from build123d import *

# Parameters (mm, degrees)
CROQUIS1_W              = 60
CROQUIS1_H              = 120
SALIENTE_EXTRUIR1_DEPTH = 50
CROQUIS2_R              = 11
SALIENTE_EXTRUIR2_DEPTH = 8
CROQUIS3_R              = 10
CORTAR_EXTRUIR1_DEPTH   = 0.1
SALIENTE_EXTRUIR3_DEPTH = 0.1
CROQUIS5_R              = 5.530403268
CROQUIS5_R_2            = 4.15467208
SALIENTE_EXTRUIR4_DEPTH = 0.1
REDONDEO1_R             = 2
CROQUIS6_R              = 9
SALIENTE_EXTRUIR5_DEPTH = 10
CHAFL_N1_SIZE           = 3
CHAFL_N1_SIZE2          = 2.100622615
CROQUIS8_R              = 6.899377385


with BuildPart() as part:
    # Croquis1 → Saliente-Extruir1 (new body)
    with BuildSketch(Plane.XY):
        with Locations((30, 60)):
            Rectangle(CROQUIS1_W, CROQUIS1_H)
    extrude(amount=SALIENTE_EXTRUIR1_DEPTH)

    # Croquis2 → Saliente-Extruir2 (add)
    with BuildSketch(Plane.XY.offset(50)):
        with Locations(Location((30, 60, 0), (0, 0, 180))):
            Circle(CROQUIS2_R)
        with Locations(Location((30, 90, 0), (0, 0, 180))):
            Circle(CROQUIS2_R)
        with Locations(Location((30, 30, 0), (0, 0, 180))):
            Circle(CROQUIS2_R)
    extrude(amount=SALIENTE_EXTRUIR2_DEPTH)

    # Croquis3 → Cortar-Extruir1 (cut)
    with BuildSketch(Plane.XY.offset(58)):
        with Locations((30, 90)):
            Circle(CROQUIS3_R)
        with Locations((30, 60)):
            Circle(CROQUIS3_R)
        with Locations((30, 30)):
            Circle(CROQUIS3_R)
    extrude(amount=-CORTAR_EXTRUIR1_DEPTH, mode=Mode.SUBTRACT)

    # Croquis4 → Saliente-Extruir3 (add)
    with BuildSketch(Plane.XY.offset(57.9)):
        Polygon((29.277033543, 82.393028635), (31.097592421, 82.393028635), (31.097592421, 93.369086775), (32.121534281, 93.369086775), (31.097592421, 94.393028635), (30.187312982, 95.303308074), (29.277033543, 94.393028635), (28.253091683, 93.369086775), (29.277033543, 93.369086775), align=None)
        Polygon((29.277033543, 26.630913225), (28.253091683, 26.630913225), (29.277033543, 25.606971365), (30.187312982, 24.696691926), (31.097592421, 25.606971365), (32.121534281, 26.630913225), (31.097592421, 26.630913225), (31.097592421, 37.606971365), (29.277033543, 37.606971365), align=None)
    extrude(amount=SALIENTE_EXTRUIR3_DEPTH)

    # Croquis5 → Saliente-Extruir4 (add)
    with BuildSketch(Plane.XY.offset(57.9)):
        with Locations((30, 60)):
            Circle(CROQUIS5_R)
        with Locations((30, 60)):
            Circle(CROQUIS5_R_2, mode=Mode.SUBTRACT)
    extrude(amount=SALIENTE_EXTRUIR4_DEPTH)

    # Redondeo1
    redondeo1_edges = [part.edges().sort_by_distance(p)[0] for p in [
        (60, 60, 50),
        (30, 120, 50),
        (0, 60, 50),
        (30, 0, 50),
        (0, 120, 25),
        (60, 120, 25),
        (60, 0, 25),
        (0, 0, 25),
    ]]
    fillet(redondeo1_edges, radius=REDONDEO1_R)

    # Croquis6 → Saliente-Extruir5 (add)
    with BuildSketch(Plane.XZ):
        with Locations(Location((30, 24, 0), (0, 0, 90))):
            Circle(CROQUIS6_R)
    extrude(amount=SALIENTE_EXTRUIR5_DEPTH)

    # Chaflán1
    chafl_n1_edges = [part.edges().sort_by_distance(p)[0] for p in [
        (30, -10, 15),
    ]]
    chafl_n1_side = [part.faces().sort_by_distance(p)[0] for p in [
        (30, -5, 15),
    ]]
    chamfer(chafl_n1_edges, length=CHAFL_N1_SIZE, length2=CHAFL_N1_SIZE2, reference=chafl_n1_side[0])

    # Barrer1: sweep along a curve in space
    with BuildLine() as barrer1_path:
        Line((30, -10, 24), (30, -18, 24))
        ThreePointArc((30, -18, 24), (33.514718626, -26.485281374, 24), (42, -30, 24))
        Line((42, -30, 24), (108, -30, 24))
        ThreePointArc((108, -30, 24), (116.485281374, -30, 20.485281374), (120, -30, 12))
        Line((120, -30, 12), (120, -30, -6))
    # Croquis8 → Barrer1 (sweep)
    with BuildSketch(Plane.XZ.offset(10)):
        with Locations((30, 24)):
            Circle(CROQUIS8_R)
    sweep(path=barrer1_path.line)


solid = part.part
Read the model definition and answer for the solid it produces. Units are mm, in the model's axes. A direction names the side the tool comes from. Round coordinates to 2 decimals unless told otherwise and drop trailing zeros. Write each loop counter-clockwise with the first axis right and the second up, starting at its lowest first coordinate (ties: lowest second). Pieces come first, ordered by that corner, then holes. Notation, with made-up numbers: (15.25, 36) - (63.25, 36) arc R10 cw to (63.25, 49) - close; hole circle Ø6 at (-14, 33). An arc over 180 degrees is marked (long way). Use a Markdown table: item, result.
(1) The part is cut by section D-D (y = 90). Write down the section's boundary in (x, z).
Reported:
| item | result |
|---|---|
| outline | (0, 0) - (60, 0) - (60, 48) arc R2 ccw to (58, 50) - (41, 50) - (41, 58) - (40, 58) - (40, 57.9) - (31.1, 57.9) - (31.1, 58) - (29.28, 58) - (29.28, 57.9) - (20, 57.9) - (20, 58) - (19, 58) - (19, 50) - (2, 50) arc R2 ccw to (0, 48) - close |
(2) Straight lines are drawn through the part: line 1 along Y through (x, z) = (30, 57); line 2 along Y through (x, z) = (13, 21); line 3 along Z through (x, y) = (58, 74). For each, find the intervals that lie inside material, in ascending order. Write a range as [from, to].
Reported:
| item | result |
|---|---|
| line 1 | [19, 41], [49, 71], [79, 101] |
| line 2 | [0, 120] |
| line 3 | [0, 50] |
(3) Which of the six approach directions +Z, -Z, +X, -X, +Y, -Y give full straight-line access (tool end or side, diameter ignored) to faces 3 (the cylindrical face through (75.462, -36.893, 24.303)), 4 (the cylindrical face through (124.66, -35.09, 2.87)), 5 (the cylindrical face through (31.432, 79.094, 53.944))?
Reported:
| item | result |
|---|---|
| face 3 | none |
| face 4 | -Z |
| face 5 | +Z |
(4) The part is cut by section C-C (x = 102.5). Write down the section's boundary in (y, z), then the cut area to 3 significant figures.
Reported:
| item | result |
|---|---|
| outline | circle Ø13.8 at (-30, 24) |
| area | 150 mm2 |
(5) The mould has two halves that part along Y. Classify faces 1 (the cylindrical face through (31.432, 49.094, 53.944)), 2 (the flat face through (30, 120, 24)): released by +Y, released by -Y, zero draft, split by the parting line, or undercut.
Reported:
| item | result |
|---|---|
| face 1 | undercut |
| face 2 | released by +Y |
(6) The part is cut by section B-B (z = 46). Write down the section's boundary in (x, y).
Reported:
| item | result |
|---|---|
| outline | (0, 2) arc R2 ccw to (2, 0) - (58, 0) arc R2 ccw to (60, 2) - (60, 118) arc R2 ccw to (58, 120) - (2, 120) arc R2 ccw to (0, 118) - close |
(7) Each of these flat-tipped pins is pushed along its axis until it touches: pin 1 Ø12 at (x, y) = (15.5, 97.5) entering from -Z; pin 2 Ø1 at (x, y) = (21.5, 13.5) entering from +Z; pin 3 Ø10 at (x, z) = (66, 25.5) entering from +Y; pin 4 Ø16 at (x, y) = (25.5, 31) entering from +Z. Where does it stop, or does it pass through?
Reported:
| item | result |
|---|---|
| pin 1 | z = 0 |
| pin 2 | z = 50 |
| pin 3 | y = -23.1 |
| pin 4 | z = 58 |
(8) The part is cut by section A-A (y = 60). Write down the section's boundary in (x, z), then the cut area to 3 significant figures.
Reported:
| item | result |
|---|---|
| outline | (0, 0) - (60, 0) - (60, 48) arc R2 ccw to (58, 50) - (41, 50) - (41, 58) - (40, 58) - (40, 57.9) - (35.53, 57.9) - (35.53, 58) - (34.15, 58) - (34.15, 57.9) - (25.85, 57.9) - (25.85, 58) - (24.47, 58) - (24.47, 57.9) - (20, 57.9) - (20, 58) - (19, 58) - (19, 50) - (2, 50) arc R2 ccw to (0, 48) - close |
| area | 3,170 mm2 |
